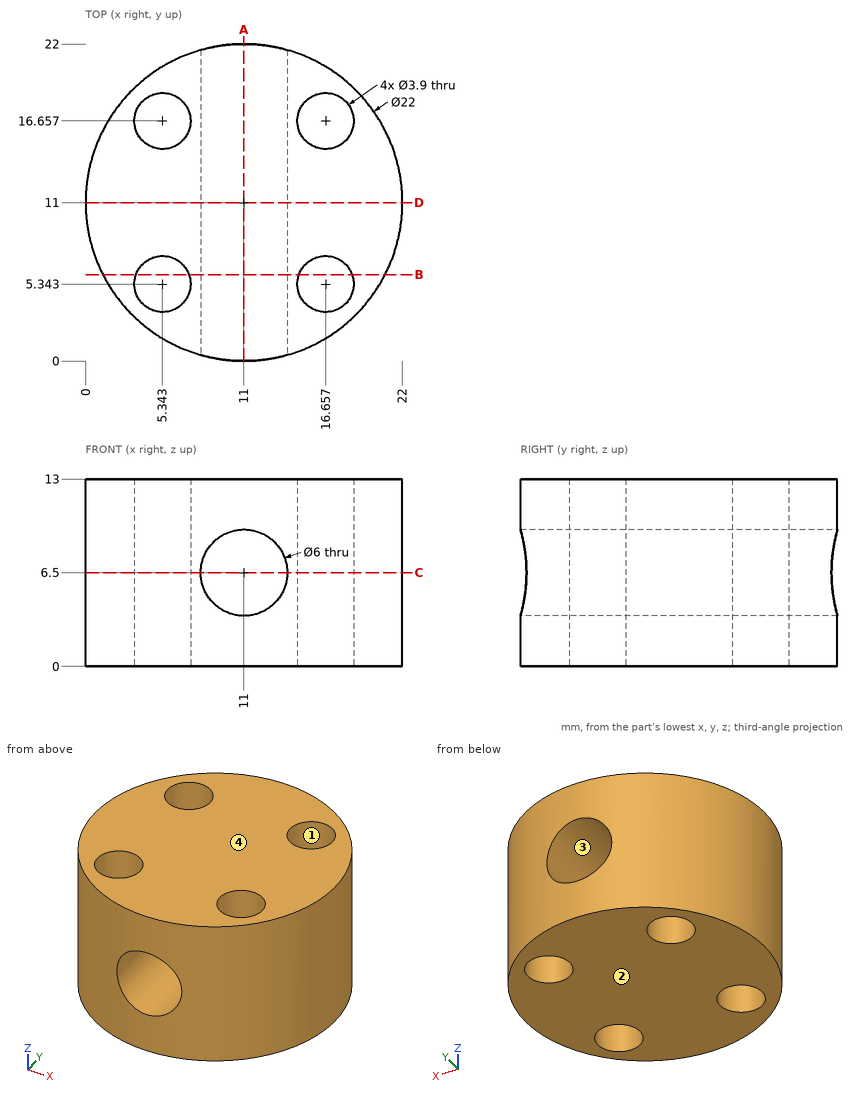
Here's the drawing with two shaded views (mm, measured from the low corner). I have some questions. Give positions to 0.01 mm unless a question says otherwise; leave off trailing zeros. Loops run counter-clockwise (first coordinate to the right, second up) from the corner with the lowest first, then second, coordinate; pieces in that order, holes last. Notation, with made-up numbers: M 33.25,71.5 L 75.25,71.5 A12 ccw 75.25,77.5 Z; hole C 32,-36 d8. An arc over 180 degrees is marked long. Answer in a Markdown table with one row per item.
1. Thinking about a two-plate mould opening in Z: for the marked faces 1, 2, 3 and 4, which applies, released by +Z, released by -Z, zero draft, split by the parting line, or undercut?
Taken from the geometry:
| item | result |
|---|---|
| face 1 | zero draft |
| face 2 | released by -Z |
| face 3 | undercut |
| face 4 | released by +Z |
2. Suppose I cut it at A-A on x = 11. Write out the boundary of the cut face in (y, z).
Taken from the geometry:
| item | result |
|---|---|
| outline | M 0,0 L 22,0 L 22,3.5 L 0,3.5 Z; M 0,9.5 L 22,9.5 L 22,13 L 0,13 Z |
3. For pin 1 Ø6 at (x, z) = (19, 3.5) entering from +Y; pin 2 Ø5 at (x, y) = (5.34, 16.66) entering from -Z; pin 3 Ø2 at (y, z) = (9, 6.5) entering from -X; pin 4 Ø3.5 at (x, y) = (16.66, 16.66) entering from +Z, each with a flat end and sliding along its axis, tell me the tip position at first contact or that it passes through.
Taken from the geometry:
| item | result |
|---|---|
| pin 1 | stops at y = 20.8 |
| pin 2 | stops at z = 0 |
| pin 3 | stops at x = 0.05 |
| pin 4 | passes through |
4. If I drill on line 1 along Y through (x, z) = (5, 11.5); line 2 along X through (y, z) = (6.25, 7.25) (1 decimal); line 3 along X through (y, z) = (5.75, 7.5), over which ranges is the centre line in solid material (lowest first)?
Taken from the geometry:
| item | result |
|---|---|
| line 1 | y = 1.78 to 3.42, 7.26 to 14.74, 18.58 to 20.22 |
| line 2 | x = 1.1 to 3.6, 7.1 to 8.1, 13.9 to 14.9, 18.4 to 20.9 |
| line 3 | x = 1.33 to 3.44, 7.25 to 8.17, 13.83 to 14.75, 18.56 to 20.67 |
5. Suppose I cut it at C-C on z = 6.5. Write out the boundary of the cut face in (x, y), plus the area to 3 significant figures.
Taken from the geometry:
| item | result |
|---|---|
| outline | M 8,0.42 L 8,21.58 A11 ccw Z; M 14,0.42 A11 ccw 14,21.58 Z; hole C 5.34,5.34 d3.9; hole C 5.34,16.66 d3.9; hole C 16.66,5.34 d3.9; hole C 16.66,16.66 d3.9 |
| area | 202 mm² |
6. Suppose I cut it at D-D on y = 11. Write out the boundary of the cut face in (x, z).
Taken from the geometry:
| item | result |
|---|---|
| outline | M 0,0 L 22,0 L 22,13 L 0,13 Z; hole C 11,6.5 d6 |
7. Suppose I cut it at B-B on y = 6. Write out the boundary of the cut face in (x, z).
Taken from the geometry:
| item | result |
|---|---|
| outline | M 1.2,0 L 3.51,0 L 3.51,13 L 1.2,13 Z; M 7.18,0 L 14.82,0 L 14.82,13 L 7.18,13 Z; M 18.49,0 L 20.8,0 L 20.8,13 L 18.49,13 Z; hole C 11,6.5 d6 |
